The drawing under review shows one solid part. Ordinate dimensions are in mm from its lowest x, y, z. A direction names the side the tool comes from. Coordinates: 2 decimals unless noted, no trailing zeros. Loops run counter-clockwise (first coordinate to the right, second up) from the corner with the lowest first, then second, coordinate; pieces in that order, holes last. Notation, with made-up numbers: (84.25, 36) - (130.25, 36) arc R24 ccw to (130.25, 68) - close; hole circle Ø8 at (-36.5, 42.25). An arc over 180 degrees is marked (long way). Answer as a JSON object with one key per item and string values. Group by question number.
Item 1: We need section C-C (x = 19). Give the boundary of the cut face in (y, z), then the cut area to 3 significant figures.
Item 2: We need section D-D (y = 4). Give the boundary of the cut face in (x, z).
Item 3: Mouldability with a two-part tool opening along Z and no side actions: class the marked faces 4, 5, 6 and 7 as released by +Z, released by -Z, zero draft, split by the parting line, or undercut.
Item 4: Tool access review of the marked faces 1, 2 and 3: name each direction out of +Z, -Z, +X, -X, +Y, -Y from which nothing blocks a thin tool from reaching the whole face with its end or side.
Item 5: We need section B-B (z = 18). Give the boundary of the cut face in (x, y), then the cut area to 3 significant figures.
Item 6: To check wall thickness, follow line 1 (X direction, y = 9.5, z = 37); line 2 (X direction, y = 14.75, z = 42). State the ranges of each line that lie inside material, in increasing order.
Item 7: Clearance check with flat-ended pins moving along their axes: pin 1 (1.5 mm diameter, centred on x = 35.5, y = 9, fed in from -Z); pin 2 (11 mm diameter, centred on x = 9, z = 16, fed in from -Y); pin 3 (10 mm diameter, centred on y = 4.5, z = 31.5, fed in from -X); pin 4 (12 mm diameter, centred on y = 20.5, z = 37.5, fed in from -X) (1 decimal). State where each tip first meets the part, or that it passes through.
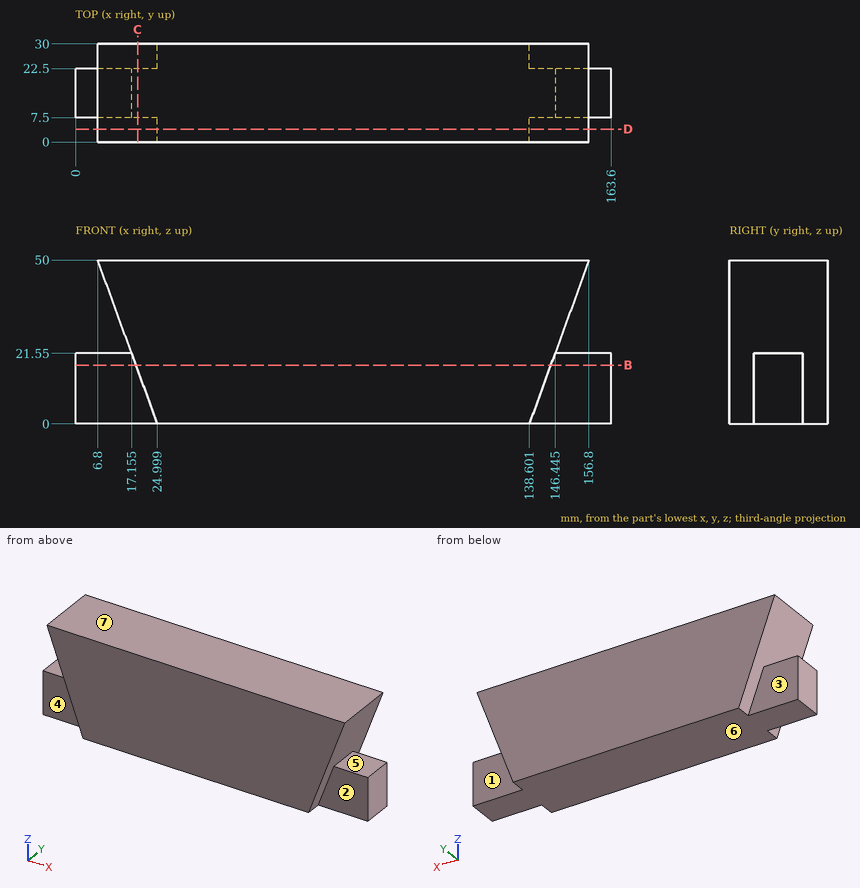
Check sheet entries:
{
 "1": {"outline": "(0, 16.48) - (7.5, 16.48) - (7.5, 0) - (22.5, 0) - (22.5, 16.48) - (30, 16.48) - (30, 50) - (0, 50) - close", "area": "1,250 mm2"},
 "2": {"outline": "(6.8, 50) - (25, 0) - (138.6, 0) - (156.8, 50) - close"},
 "3": {"face 4": "zero draft", "face 5": "undercut", "face 6": "released by -Z", "face 7": "released by +Z"},
 "4": {"face 1": "-Z, +X, +Y", "face 2": "-Z, +X, -Y", "face 3": "-Z, -X, +Y"},
 "5": {"outline": "(0, 7.5) - (18.45, 7.5) - (18.45, 0) - (145.15, 0) - (145.15, 7.5) - (163.6, 7.5) - (163.6, 22.5) - (145.15, 22.5) - (145.15, 30) - (18.45, 30) - (18.45, 22.5) - (0, 22.5) - close", "area": "4,350 mm2"},
 "6": {"line 1": "x = 11.53 to 152.07", "line 2": "x = 9.71 to 153.89"},
 "7": {"pin 1": "stops at z = 0", "pin 2": "stops at y = 7.5", "pin 3": "stops at x = 11.71", "pin 4": "stops at x = 9.2"}
}
